Can you work these out from the model? Positions are in its coordinate system, mm. A direction names the side the tool comes from. Give positions to 0.01 mm unless a question says otherwise; leave off trailing zeros. Loops run counter-clockwise (first coordinate to the right, second up) from the corner with the lowest first, then second, coordinate; pieces in that order, holes last. Notation, with made-up numbers: (-39.5, -14) -> (-2.5, -14) arc R20 cw to (-2.5, 23) -> close; hole circle Ø3 at (57.5, 33.5). An arc over 180 degrees is marked (long way). Return JSON: item names as keys, results as strings. Group by question number.
Q1. Will these pins go through, and if not, where does the flat tip stop? pin 1 (5 mm diameter, centred on x = -17, z = 69.5, fed in from +Y) (3 decimals); pin 2 (8 mm diameter, centred on y = 18.5, z = 47.5, fed in from -X) (3 decimals).
Q2. I need wall thicknesses on line 1 along Y through (x, z) = (-1.4, 44.45) (3 decimals); line 2 along X through (y, z) = (15, 68.5) (3 decimals); line 3 along Y through (x, z) = (-23.25, 76.5) (3 decimals). Which ranges of each line are inside material? Lowest first, please. Write a range as [from, to].
Q3. Which directions (+Z, -Z, +X, -X, +Y, -Y) give clear straight access to the entire face, cutting with the end or side of a thin tool? Please do faces 5 (the flat face through (-1.61, 7.37, 9.57)), 6 (the flat face through (-14, 3.175, 44)), 7 (the flat face through (-13, 0, 44)).
Q4. Suppose I cut it at B-B, the plane y = 7.5. Please give me the cut outline in (x, z) (3 decimals).
Q5. Suppose I cut it at D-D, the plane y = 21.75. Please give me the cut outline in (x, z) (3 decimals).
Q6. Suppose I cut it at C-C, the plane x = -19. Please give me the cut outline in (y, z) (3 decimals), and give its area (3 significant figures).
Q7. Suppose I cut it at A-A, the plane z = 44.45. Please give me the cut outline in (x, y) (3 decimals).
Q8. Thinking about a two-plate mould opening in Y: for faces 1 (the flat face through (-25.4, 2, 44)), 2 (the cylindrical face through (-1.61, 12.738, 24.116)), 3 (the flat face through (-7.37, 1.61, 79.42)), 4 (the cylindrical face through (-1.61, 13.32, 43.19)), which applies, pulls with the +Y half, pulls with the -Y half, needs draft (parallel to the pull), parting line crosses it, or undercut?
```python
from build123d import *

# Parameters (mm, degrees)
BOSS_EXTRUDE1_DEPTH     = 88.9
SKETCH2_W               = 6.35
SKETCH2_H               = 6.35
CUT_EXTRUDE4_DEPTH      = 18.960512242
CUT_EXTRUDE4_DEPTH_BACK = 18.960512242
SKETCH3_R               = 1.5875
CUT_EXTRUDE5_DEPTH      = 4.175


with BuildPart() as part:
    # Sketch1 → Boss-Extrude1 (new body)
    with BuildSketch(Plane.XY):
        Polygon((0, 0), (0, 25.4), (-3.175, 25.4), (-3.175, 3.175), (-25.4, 3.175), (-25.4, 0), align=None)
    extrude(amount=BOSS_EXTRUDE1_DEPTH)

    # Sketch2 → Cut-Extrude4 (cut, two sides)
    with BuildSketch(Plane(origin=(0, 0, 0), x_dir=(0, 0, -1), z_dir=(0.707106781, 0.707106781, 0))) as cut_extrude4_sk:
        with Locations((-79.375, 3.175)):
            Rectangle(SKETCH2_W, SKETCH2_H)
        with Locations((-9.525, 3.175)):
            Rectangle(SKETCH2_W, SKETCH2_H)
    extrude(amount=CUT_EXTRUDE4_DEPTH, mode=Mode.SUBTRACT)
    extrude(cut_extrude4_sk.sketch, amount=-CUT_EXTRUDE4_DEPTH_BACK, mode=Mode.SUBTRACT)

    # Sketch3 → Cut-Extrude5 (cut, through all)
    with BuildSketch(Plane.ZY.offset(3.175)):
        with Locations((44.45, 14.2875)):
            Circle(SKETCH3_R)
        with Locations((24.4602, 14.2875)):
            Circle(SKETCH3_R)
        with Locations((64.4398, 14.2875)):
            Circle(SKETCH3_R)
    extrude(amount=-CUT_EXTRUDE5_DEPTH, mode=Mode.SUBTRACT)


solid = part.part
```
Ans:
{
 "1": {"pin 1": "stops at y = 3.175", "pin 2": "stops at x = -3.175"},
 "2": {"line 1": "y = [0, 12.7], [15.875, 25.4]", "line 2": "x = [-3.175, 0]", "line 3": "y = [0, 3.175]"},
 "3": {"face 5": "+X, -Y", "face 6": "+Z, -Z, -X, +Y", "face 7": "+Z, -Z, +X, -X, -Y"},
 "4": {"outline": "(-3.175, 0) -> (0, 0) -> (0, 6.35) -> (-1.48, 6.35) -> (-1.48, 12.7) -> (0, 12.7) -> (0, 76.2) -> (-1.48, 76.2) -> (-1.48, 82.55) -> (0, 82.55) -> (0, 88.9) -> (-3.175, 88.9) -> close"},
 "5": {"outline": "(-3.175, 0) -> (0, 0) -> (0, 88.9) -> (-3.175, 88.9) -> close"},
 "6": {"outline": "(0, 0) -> (3.175, 0) -> (3.175, 88.9) -> (0, 88.9) -> close", "area": "282 mm^2"},
 "7": {"outline": "(-25.4, 0) -> (0, 0) -> (0, 12.7) -> (-3.175, 12.7) -> (-3.175, 3.175) -> (-25.4, 3.175) -> close; (-3.175, 15.875) -> (0, 15.875) -> (0, 25.4) -> (-3.175, 25.4) -> close"},
 "8": {"face 1": "needs draft", "face 2": "undercut", "face 3": "pulls with the -Y half", "face 4": "undercut"}
}
